Check sheet for the modelled part. Datum: model origin and axes. Units: mm. A direction names the side the tool comes from. Coordinates: 2 decimals unless noted, no trailing zeros. Loops run counter-clockwise (first coordinate to the right, second up) from the corner with the lowest first, then second, coordinate; pieces in that order, holes last. Notation, with made-up numbers: (79, 60.5) - (83, 60.5) arc R22 cw to (83, 88.5) - close; hole circle Ø2 at (59, 1.5). An arc over 180 degrees is marked (long way). Use a Markdown table: item, result. Add a question column.
1) Sectioned sample at B-B, the plane x = -13. Enter the section's corners in (y, z) (3 decimals), then the cut area to 3 significant figures.
2) Sectioned sample at A-A, the plane z = 1.25. Enter the section's corners in (x, y) (3 decimals), then the cut area to 3 significant figures.
3) Go/stop test with flat-tipped pins: P1, Ø1.5, axis at y = 0, z = 1, coming from the -X side (3 decimals); P2, Ø12, axis at x = 13.5, y = 13, coming from the +Z side; P3, Ø3, axis at y = 21, z = 4, coming from the +X side. Record where each tip stops, or that it passes through.
4) Tool access check on faces 1 (the cylindrical face through (-24.676, -4.011, 1.479)), 2 (the flat face through (-9.25, 12.29, 1.48)), 3 (the flat face through (9.04, 10.2, 1.52)). Record the directions out of +Z, -Z, +X, -X, +Y, -Y that give a thin tool (end or side, any length) a straight path to the whole face; none if there is none.
5) Sectioned sample at C-C, the plane z = 5.75. Enter the section's corners in (x, y) (3 decimals).
6) Draft check along Y on faces 4 (the flat face through (5, 21, 3)), 5 (the flat face through (0, 1.525, 3)), 6 (the flat face through (-12, -5.525, 1)). Enter one of: pulls with the +Y half, pulls with the -Y half, needs draft (parallel to the pull), parting line crosses it, or undercut.
7) Thickness scan on line 1 (Y direction, x = 0.5, z = 1.75) (3 decimals); line 2 (Z direction, x = 15.5, y = 13); line 3 (Y direction, x = -7.5, z = 2.5) (3 decimals). Record the ranges inside material, lowest first.
8) Sectioned sample at D-D, the plane x = 8. Enter the section's corners in (y, z), then the cut area to 3 significant figures.
from build123d import *
from build123d.topology import SkipClean

# Parameters (mm, degrees)
BOSS_EXTRUDE2_DEPTH = 3
CUT_EXTRUDE1_DEPTH  = 3
BOSS_EXTRUDE3_DEPTH = 4
FILLET1_R           = 2


with BuildPart() as part:
    # Sketch1 → Boss-Extrude2 (new body)
    with BuildSketch(Plane.XY):
        with BuildLine():
            ThreePointArc((0, -5.525), (-2.878801834, -4.715731651), (-4.91426495, -2.525))
            Line((-4.91426495, -2.525), (-24.872160642, -2.525))
            ThreePointArc((-24.872160642, -2.525), (-24.672642191, -4.032459214), (-24.381845193, -5.525))
            Line((-24.381845193, -5.525), (0, -5.525))
        make_face()
        with BuildLine():
            ThreePointArc((0, -2.525), (1.123610253, -2.261222015), (2.01246118, -1.525))
            Line((2.01246118, -1.525), (-2.01246118, -1.525))
            ThreePointArc((-2.01246118, -1.525), (-1.123610253, -2.261222015), (0, -2.525))
        make_face()
        with BuildLine():
            ThreePointArc((2.01246118, 1.525), (0, 2.525), (-2.01246118, 1.525))
            Line((-2.01246118, 1.525), (2.01246118, 1.525))
        make_face()
        with BuildLine():
            Line((-3.728656931, 4.077099765), (-2.01246118, 1.525))
            ThreePointArc((-2.01246118, 1.525), (0, 2.525), (2.01246118, 1.525))
            Line((2.01246118, 1.525), (4.61980513, 3.030350732))
            ThreePointArc((4.61980513, 3.030350732), (0.687355194, 5.482076964), (-3.728656931, 4.077099765))
        make_face()
        with BuildLine():
            ThreePointArc((0, -2.525), (-1.123610253, -2.261222015), (-2.01246118, -1.525))
            ThreePointArc((-2.01246118, -1.525), (-2.525, 0), (-2.01246118, 1.525))
            Line((-2.01246118, 1.525), (-3.728656931, 4.077099765))
            ThreePointArc((-3.728656931, 4.077099765), (-5.438010205, 0.976560297), (-4.91426495, -2.525))
            Line((-4.91426495, -2.525), (0, -2.525))
        make_face()
        with BuildLine():
            Line((0, -5.525), (0, -2.525))
            Line((0, -2.525), (-4.91426495, -2.525))
            ThreePointArc((-4.91426495, -2.525), (-2.878801834, -4.715731651), (0, -5.525))
        make_face()
        with BuildLine():
            ThreePointArc((2.525, 0), (2.39343785, -0.804412991), (2.01246118, -1.525))
            ThreePointArc((2.01246118, -1.525), (1.123610253, -2.261222015), (0, -2.525))
            Line((0, -2.525), (0, -5.525))
            ThreePointArc((0, -5.525), (3.906764966, -3.906764966), (5.525, 0))
            Line((5.525, 0), (2.525, 0))
        make_face()
        with BuildLine():
            ThreePointArc((2.01246118, 1.525), (2.39343785, 0.804412991), (2.525, 0))
            Line((2.525, 0), (5.525, 0))
            ThreePointArc((5.525, 0), (5.293866656, 1.581328817), (4.61980513, 3.030350732))
            Line((4.61980513, 3.030350732), (2.01246118, 1.525))
        make_face()
        with BuildLine():
            Line((-14.622794466, 20.277422963), (-3.728656931, 4.077099765))
            ThreePointArc((-3.728656931, 4.077099765), (0.687355194, 5.482076964), (4.61980513, 3.030350732))
            Line((4.61980513, 3.030350732), (21.491693232, 12.771339869))
            ThreePointArc((21.491693232, 12.771339869), (5.087313969, 24.476912317), (-14.622794466, 20.277422963))
        make_face()
    extrude(amount=BOSS_EXTRUDE2_DEPTH)

    # Sketch2 → Cut-Extrude1 (cut)
    with BuildSketch(Plane.XY.offset(3)):
        with BuildLine():
            Line((-8.943662301, 19.000286962), (-0.824328522, 6.926285605))
            Line((-0.824328522, 6.926285605), (2.61980513, 6.494452347))
            Line((2.61980513, 6.494452347), (15.641340759, 14.012439447))
            ThreePointArc((15.641340759, 14.012439447), (4.175449663, 20.580709903), (-8.943662301, 19.000286962))
        make_face()
    extrude(amount=-CUT_EXTRUDE1_DEPTH, mode=Mode.SUBTRACT)

    # Sketch3 → Boss-Extrude3 (add)
    with SkipClean():  # the faces are left unmerged after this step: merging them gives an invalid solid
        with BuildSketch(Plane.XY.offset(3)):
            with BuildLine():
                ThreePointArc((5.525, 0), (5.293866656, 1.581328817), (4.61980513, 3.030350732))
                ThreePointArc((4.61980513, 3.030350732), (0.687355194, 5.482076964), (-3.728656931, 4.077099765))
                ThreePointArc((-3.728656931, 4.077099765), (-5.438010205, 0.976560297), (-4.91426495, -2.525))
                ThreePointArc((-4.91426495, -2.525), (-2.878801834, -4.715731651), (0, -5.525))
                ThreePointArc((0, -5.525), (3.906764966, -3.906764966), (5.525, 0))
            make_face()
            with BuildLine():
                Line((-2.01246118, 1.525), (2.01246118, 1.525))
                ThreePointArc((2.01246118, 1.525), (2.525, 0), (2.01246118, -1.525))
                Line((2.01246118, -1.525), (-2.01246118, -1.525))
                ThreePointArc((-2.01246118, -1.525), (-2.525, 0), (-2.01246118, 1.525))
            make_face(mode=Mode.SUBTRACT)
        extrude(amount=BOSS_EXTRUDE3_DEPTH)

    # Fillet1
    fillet1_edges = [part.edges().sort_by_distance(p)[0] for p in [
        (3.728656931, -4.077099765, 7),
    ]]
    fillet(fillet1_edges, radius=FILLET1_R)


solid = part.part
Solved:
| question | item | result |
|---|---|---|
| 1 | outline | (-5.525, 0) - (-2.525, 0) - (-2.525, 3) - (-5.525, 3) - close; (17.864, 0) - (21.354, 0) - (21.354, 3) - (17.864, 3) - close |
| 1 | area | 19.5 mm2 |
| 2 | outline | (-24.872, -2.525) arc R25 ccw to (-24.382, -5.525) - (0, -5.525) arc R5.525 ccw to (4.62, 3.03) - (21.492, 12.771) arc R25 ccw to (-14.623, 20.277) - (-3.729, 4.077) arc R5.525 ccw to (-4.914, -2.525) - close; hole (-8.944, 19) - (-0.824, 6.926) - (2.62, 6.494) - (15.641, 14.012) arc R21 ccw to start; hole (-2.012, -1.525) - (2.012, -1.525) arc R2.525 ccw to (2.012, 1.525) - (-2.012, 1.525) arc R2.525 ccw to start |
| 2 | area | 427 mm2 |
| 3 | P1 | stops at x = -5.525 |
| 3 | P2 | stops at z = 3 |
| 3 | P3 | stops at x = 15.16 |
| 4 | face 1 | +Z, -Z, -X, -Y |
| 4 | face 2 | +Z, -Z, -X |
| 4 | face 3 | +Z, -Z |
| 5 | outline | circle Ø10.758 at (0, 0); hole (-2.012, -1.525) - (2.012, -1.525) arc R2.525 ccw to (2.012, 1.525) - (-2.012, 1.525) arc R2.525 ccw to start |
| 6 | face 4 | needs draft |
| 6 | face 5 | undercut |
| 6 | face 6 | pulls with the -Y half |
| 7 | line 1 | y = -5.502 to -1.525, 1.525 to 6.76, 20.994 to 24.995 |
| 7 | line 2 | z = 0 to 3 |
| 7 | line 3 | y = -5.525 to -2.525, 9.685 to 16.853, 19.615 to 23.848 |
| 8 | outline | (4.98, 0) - (9.6, 0) - (9.6, 3) - (4.98, 3) - close; (19.42, 0) - (23.69, 0) - (23.69, 3) - (19.42, 3) - close |
| 8 | area | 26.7 mm2 |
